Check sheet for the modelled part. Datum: model origin and axes. Units: mm. Give positions to 0.01 mm unless a question says otherwise; leave off trailing zeros. Order: outer loops, then holes, each group sorted by start corner. A loop starts at its lowest first (then second) coordinate and runs counter-clockwise, first axis right, second up.
Item 1: Material ranges on line 1 along X through (y, z) = (0, 8); line 2 along X through (y, z) = (11, 2.25); line 3 along Y through (x, z) = (10.5, 7), recorded low to high.
Item 2: Sectioned sample at D-D on x = 0. Record the boundary of the cut face in (y, z), and give its area (3 significant figures).
Item 3: Sectioned sample at B-B on z = 9.25. Record the boundary of the cut face in (x, y), and give its area (3 significant figures).
Item 4: Gauge pin test, flat ends, axial feed: P1, Ø1.5, axis at y = -1.5, z = 6.5, coming from the +X side; P2, Ø1.5, axis at y = -2.5, z = 2, coming from the -X side; P3, Ø2, axis at y = 11.5, z = 4.5, coming from the -X side. Record the tip position at first contact, or that the pin passes through.
Item 5: Sectioned sample at A-A on y = 0. Record the boundary of the cut face in (x, z), and give its area (3 significant figures).
Item 6: Sectioned sample at C-C on y = 5.5. Record the boundary of the cut face in (x, z).
from build123d import *

# Parameters (mm, degrees)
PAD_DEPTH = 10
FILLET_R  = 0.75


with BuildPart() as part:
    # Sketch → Pad (new body)
    with BuildSketch(Plane.XY):
        with BuildLine():
            ThreePointArc((8.603647, -12.287281), (0, 15), (-8.603647, -12.287281))
            Line((-7.456494, -10.648977), (-8.603647, -12.287281))
            ThreePointArc((7.456494, -10.648977), (0, 13), (-7.456494, -10.648977))
            Line((8.603647, -12.287281), (7.456494, -10.648977))
        make_face()
    extrude(amount=PAD_DEPTH)

    # Fillet
    fillet_edges = [part.edges().sort_by_distance(p)[0] for p in [
        (7.456494, -10.648977, 5),
        (8.603647, -12.287281, 5),
        (-7.456494, -10.648977, 5),
        (-8.603647, -12.287281, 5),
    ]]
    fillet(fillet_edges, radius=FILLET_R)


solid = part.part
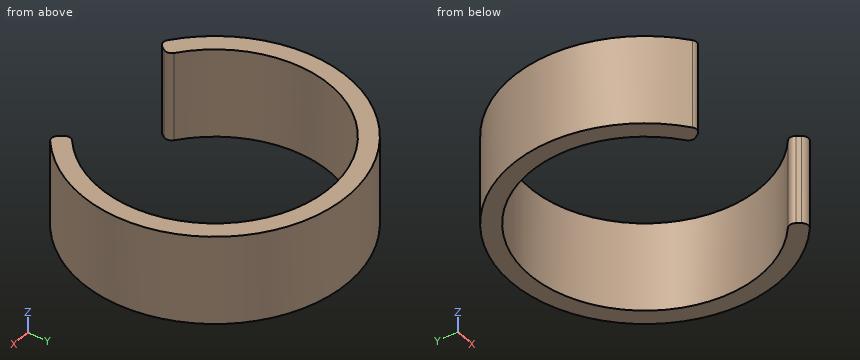
Report:
1. line 1: x = -15 to -13, 13 to 15
1. line 2: x = -10.2 to -6.93, 6.93 to 10.2
1. line 3: y = -10.71 to -7.66, 7.66 to 10.71
2. outline: (13, 0) - (15, 0) - (15, 10) - (13, 10) - close
2. area: 20.0 mm2
3. outline: (-9.24, -11.82) arc R0.75 ccw to (-8.16, -11.66) - (-7.87, -11.25) arc R0.75 ccw to (-8.03, -10.23) arc R13 cw (long way) to (8.03, -10.23) arc R0.75 ccw to (7.87, -11.25) - (8.16, -11.66) arc R0.75 ccw to (9.24, -11.82) arc R15 ccw (long way) to start
3. area: 141 mm2
4. P1: stops at x = 14.98
4. P2: stops at x = -14.9
4. P3: stops at x = -10.71
5. outline: (-15, 0) - (-13, 0) - (-13, 10) - (-15, 10) - close; (13, 0) - (15, 0) - (15, 10) - (13, 10) - close
5. area: 40.0 mm2
6. outline: (-13.96, 0) - (-11.78, 0) - (-11.78, 10) - (-13.96, 10) - close; (11.78, 0) - (13.96, 0) - (13.96, 10) - (11.78, 10) - close
